Autodesk Inventor part; units mm, degrees
ref_plane "YZ Plane" through (0, 0, 0) normal (1, 0, 0) x (0, 1, 0)
ref_plane "XZ Plane" through (0, 0, 0) normal (0, 1, 0) x (-1, 0, 0)
ref_plane "XY Plane" through (0, 0, 0) normal (0, 0, 1) x (1, 0, 0)
sketch "Skizze1" plane through (0, 0, 0) normal (0, 0, 1) x (1, 0, 0)
  line L0 (-13, -20) -> (13, -20)
  line L1 (13, -20) -> (13, 18)
  line L2 (11, 20) -> (-11, 20)
  line L3 (-13, 18) -> (-13, -20)
  line L4 (-13, -20) -> (13, 20) construction
  line L5 (13, -20) -> (-13, 20) construction
  arc A0 (13, 18) -> (11, 20) centre (11, 18) ccw
  arc A1 (-11, 20) -> (-13, 18) centre (-11, 18) ccw
  line L6 (-11, 21.8) -> (11, 21.8)
  arc A2 (14.8, 18) -> (11, 21.8) centre (11, 18) ccw
  line L7 (14.8, 18) -> (14.8, -21.8)
  line L8 (14.8, -21.8) -> (-14.8, -21.8)
  line L9 (-14.8, -21.8) -> (-14.8, 18)
  arc A3 (-11, 21.8) -> (-14.8, 18) centre (-11, 18) ccw
  line L10 (-4.25, 10) -> (4.25, 10)
  line L11 (4.25, 10) -> (4.25, 1.5)
  line L12 (4.25, 1.5) -> (-4.25, 1.5)
  line L13 (-4.25, 1.5) -> (-4.25, 10)
  circle A4 centre (0, 5.75) radius 4.25 construction
  line L14 (0, 20) -> (0, -20) construction
  circle A5 centre (0, 5.75) radius 3.75
  point P0 (0, 0)
  dimension "d0" = 26
  dimension "d7" = 2
  dimension "d8" = 1.8
  dimension "d13" = 21.5
  dimension "d14" = 8.5
  dimension "d15" = 7.5
  dimension "d16" = 40
extrude "Extrusion1" add sketch "Skizze1" against normal blind 12 contours L6 A2 L7 L8 L9 A3
extrude "Extrusion2" add sketch "Skizze1" along normal blind 1.2 contours L3 A1 L2 A0 L1 L0 | L6 A2 L7 L8 L9 A3 | L10 L11 L12 L13
sketch "Skizze2" plane through (-14.8, -21.8, -12) normal (0, -1, 0) x (1, 0, 0)
  line L0 (0, 0) -> (0, 13.2)
  line L1 (29.6, 0) -> (0, 0)
  line L2 (29.6, 0) -> (29.6, 13.2)
  line L3 (0, 13.2) -> (29.6, 13.2)
  line L4 (3.8, 0) -> (25.8, 0)
  line L5 (7.3, 0) -> (22.3, 0)
  line L6 (22.3, 0) -> (22.3, 7)
  line L7 (22.3, 7) -> (7.3, 7)
  line L8 (7.3, 7) -> (7.3, 0)
  point P0 (14.8, 12)
  point P1 (14.8, 0)
  point P2 (22.3, 0)
  dimension "d9" = 15
  dimension "d10" = 7
extrude "Extrusion3" cut sketch "Skizze2" against normal up to next contours L8 L7 L6 L1
properties part number "Camera-Cover"
Here's how the part is built. I have some questions about the finished solid (model axes, mm). A direction names the side the tool comes from. Give positions to 0.01 mm unless a question says otherwise; leave off trailing zeros. Order: outer loops, then holes, each group sorted by start corner. A loop starts at its lowest first (then second) coordinate and runs counter-clockwise, first axis right, second up. Notation, with made-up numbers: (-37.5, -10.75) -> (3.5, -10.75) arc R8 ccw to (3.5, -1.75) -> close; hole circle Ø10 at (49.5, 47). An arc over 180 degrees is marked (long way). Use a Markdown table: item, result. Add a question column.
Item 1: Imagine slicing it at A-A on x = 0. Please give me the cut outline in (y, z), plus the area to 3 significant figures.
Item 2: For faces 1 (the face through (-14.8, -2, -5)), 2 (the face through (-13, -1, -6)), 3 (the face through (0, -21, -5)), which set-ups out of +Z, -Z, +X, -X, +Y, -Y let a thin tool reach every point of the face, with its end or its side?
Item 3: I need wall thicknesses on line 1 (X direction, y = -19, z = -1); line 2 (Y direction, x = 0, z = 0.7); line 3 (Y direction, x = -5.75, z = -0.5). Which ranges of each line are inside material? Lowest first, please.
Item 4: Imagine slicing it at D-D on y = -10.5. Please give me the cut outline in (x, z).
Item 5: Imagine slicing it at B-B on y = 5.75. Please give me the cut outline in (x, z), plus the area to 3 significant figures.
Item 6: Will these pins go through, and if not, where does the flat tip stop? pin 1 (2 mm diameter, centred on x = -1.5, y = -21, fed in from -Z); pin 2 (4 mm diameter, centred on x = 1, y = -4.5, fed in from -Z).
Item 7: If we mould it in two halves opening along X, with no side actions, what happens to faces 4 (the face through (0, 20, -6)), 5 (the face through (0, 0, 1.2)), 6 (the face through (13.716, 20.657, -5.308))? For each: pulls with the +X half, pulls with the -X half, needs draft (parallel to the pull), parting line crosses it, or undercut.
Item 8: Imagine slicing it at C-C on z = 0.5. Please give me the cut outline in (x, y), plus the area to 3 significant figures.
Data:
| question | item | result |
|---|---|---|
| 1 | outline | (-21.8, -5) -> (-20, -5) -> (-20, 0) -> (2, 0) -> (2, 1.2) -> (-21.8, 1.2) -> close; (9.5, 0) -> (20, 0) -> (20, -12) -> (21.8, -12) -> (21.8, 1.2) -> (9.5, 1.2) -> close |
| 1 | area | 73.9 mm² |
| 2 | face 1 | +Z, -Z, -X, +Y, -Y |
| 2 | face 2 | -Z |
| 2 | face 3 | -Z, -Y |
| 3 | line 1 | x = -14.8 to -13, 13 to 14.8 |
| 3 | line 2 | y = -21.8 to 2, 9.5 to 21.8 |
| 3 | line 3 | y = -21.8 to -20, 20 to 21.8 |
| 4 | outline | (-14.8, -12) -> (-13, -12) -> (-13, 0) -> (13, 0) -> (13, -12) -> (14.8, -12) -> (14.8, 1.2) -> (-14.8, 1.2) -> close |
| 5 | outline | (-14.8, -12) -> (-13, -12) -> (-13, 0) -> (-3.75, 0) -> (-3.75, 1.2) -> (-14.8, 1.2) -> close; (3.75, 0) -> (13, 0) -> (13, -12) -> (14.8, -12) -> (14.8, 1.2) -> (3.75, 1.2) -> close |
| 5 | area | 69.7 mm² |
| 6 | pin 1 | stops at z = -5 |
| 6 | pin 2 | stops at z = 0 |
| 7 | face 4 | undercut |
| 7 | face 5 | needs draft |
| 7 | face 6 | pulls with the +X half |
| 8 | outline | (-14.8, -21.8) -> (14.8, -21.8) -> (14.8, 18) arc R3.8 ccw to (11, 21.8) -> (-11, 21.8) arc R3.8 ccw to (-14.8, 18) -> close; hole circle Ø7.5 at (0, 5.75) |
| 8 | area | 1,240 mm² |
